Can you work these out from the model? Positions are in its coordinate system, mm. Face numbers are marked on the shaded views. A direction names the side the tool comes from. Round coordinates to 2 decimals unless told otherwise and drop trailing zeros. Order: outer loops, then holes, each group sorted by start corner. A loop starts at its lowest first (then second) coordinate and runs counter-clockwise, first axis right, second up. Notation, with made-up numbers: M 60.5,-3.5 L 108.5,-3.5 A22 cw 108.5,35.5 Z; hole C -4.75,85.5 d8. An arc over 180 degrees is marked long. Answer as a JSON object with one key per item and string values. Group by question number.
```python
from build123d import *

# Parameters (mm, degrees)
SALIENTE_EXTRUIR1_DEPTH = 25.8
CORTAR_EXTRUIR1_REACH   = 53.135
CROQUIS2_R              = 0.986321187
CROQUIS2_W              = 18.5
CROQUIS2_H              = 11.8
CORTAR_EXTRUIR2_DEPTH   = 47.498669213


with BuildPart() as part:
    # Croquis1 → Saliente-Extruir1 (new body)
    with BuildSketch(Plane.XY):
        Polygon((-15.36468389, -0.528688711), (-15.36468389, -1.528688711), (23.08488752, -1.528688711), (23.08488752, -29.783472062), (-25.31094407, -29.783472062), (-25.31094407, -36.701823748), (-24.31094407, -36.701823748), (-24.31094407, -30.783472062), (24.08488752, -30.783472062), (24.08488752, -0.528688711), align=None)
    extrude(amount=SALIENTE_EXTRUIR1_DEPTH)

    # Croquis2 → Cortar-Extruir1 (cut, up to next)
    with BuildSketch(Plane(origin=(0, -0.528688711, 0), x_dir=(1, 0, 0), z_dir=(0, 1, 0)), mode=Mode.PRIVATE) as cortar_extruir1_sk1:
        with Locations(Location((5.43531611, -12.9, 0), (0, 0, 180))):
            Circle(CROQUIS2_R)
    cortar_extruir1_tool1 = extrude(cortar_extruir1_sk1.sketch, amount=-CORTAR_EXTRUIR1_REACH, mode=Mode.PRIVATE) & part.part
    # Croquis2 → Cortar-Extruir1 (cut, up to next)
    with BuildSketch(Plane(origin=(0, -0.528688711, 0), x_dir=(1, 0, 0), z_dir=(0, 1, 0)), mode=Mode.PRIVATE) as cortar_extruir1_sk2:
        with Locations((-6.11468389, -12.9)):
            Rectangle(CROQUIS2_W, CROQUIS2_H)
    cortar_extruir1_tool2 = extrude(cortar_extruir1_sk2.sketch, amount=-CORTAR_EXTRUIR1_REACH, mode=Mode.PRIVATE) & part.part
    add(cortar_extruir1_tool1.solids().sort_by_distance((5.435316, -0.528689, 12.9))[0], mode=Mode.SUBTRACT)
    add(cortar_extruir1_tool2.solids().sort_by_distance((-6.114684, -0.528689, 12.9))[0], mode=Mode.SUBTRACT)

    # Croquis3 → Cortar-Extruir2 (cut, through all)
    with BuildSketch(Plane(origin=(0, -29.783472062, 0), x_dir=(1, 0, 0), z_dir=(0, 1, 0))):
        with BuildLine():
            Line((-25.31094407, -1.35), (9.391397529, -1.35))
            ThreePointArc((9.391397529, -1.35), (13.99905593, -12.9), (9.391397529, -24.45))
            Line((9.391397529, -24.45), (-25.31094407, -24.45))
            Line((-25.31094407, -24.45), (-25.31094407, -1.35))
        make_face()
    extrude(amount=-CORTAR_EXTRUIR2_DEPTH, mode=Mode.SUBTRACT)


solid = part.part
```
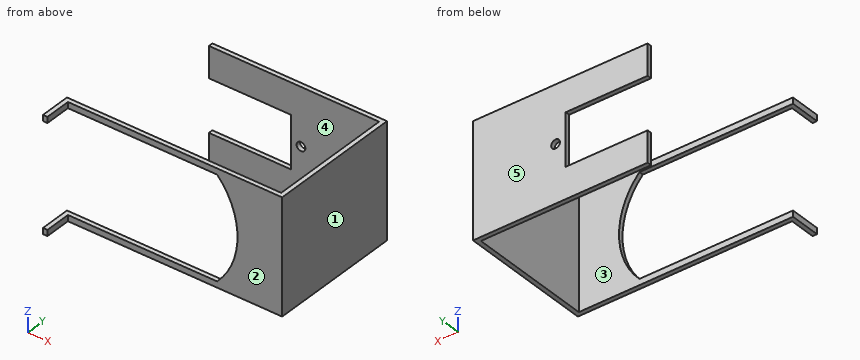
1) Which directions (+Z, -Z, +X, -X, +Y, -Y) give clear straight access to the entire face, cutting with the end or side of a thin tool? Please do the marked faces 4 and 5.
2) For pin 1 (6 mm diameter, centred on x = 6.5, z = 3, fed in from -Y); pin 2 (5.5 mm diameter, centred on x = -1.5, y = -34.5, fed in from +Z); pin 3 (0.7 mm diameter, centred on y = -34, z = 25, fed in from +X); pin 4 (0.8 mm diameter, centred on y = -1, z = 2.5, fed in from -X), each with a flat end and sliding along its axis, tell me the tip position at first contact or that it passes through.
3) If we section it at D-D on x = 12: Write out the boundary of the cut face in (y, z).
4) If we section it at C-C on x = -8.5: Write out the boundary of the cut face in (y, z).
5) I need wall thicknesses on line 1 along Y through (x, z) = (20, 14.75); line 2 along X through (y, z) = (-25, 14.5); line 3 along Y through (x, z) = (-5, 1.5). Which ranges of each line are inside material? Lowest first, please.
6) We'd pull the mould along Y, two halves only. Please class the marked faces 1, 2 and 3: +Y half, -Y half, draft (parallel to the pull), parting line (faces both ways), or undercut.
7) If we section it at A-A on z = 12.9: Write out the boundary of the cut face in (x, y), plus the area to 3 significant figures.
8) If we section it at B-B on x = 17.5: Write out the boundary of the cut face in (y, z), plus the area to 3 significant figures.
Findings:
{
 "1": {"face 4": "+Z, -Z, -X", "face 5": "+Z, -Z, +X, -X, +Y"},
 "2": {"pin 1": "stops at y = -30.78", "pin 2": "passes through", "pin 3": "stops at x = -24.31", "pin 4": "stops at x = -15.36"},
 "3": {"outline": "M -30.78,0 L -29.78,0 L -29.78,4.96 L -30.78,4.96 Z; M -30.78,20.84 L -29.78,20.84 L -29.78,25.8 L -30.78,25.8 Z; M -1.53,0 L -0.53,0 L -0.53,25.8 L -1.53,25.8 Z"},
 "4": {"outline": "M -30.78,0 L -29.78,0 L -29.78,1.35 L -30.78,1.35 Z; M -30.78,24.45 L -29.78,24.45 L -29.78,25.8 L -30.78,25.8 Z; M -1.53,0 L -0.53,0 L -0.53,7 L -1.53,7 Z; M -1.53,18.8 L -0.53,18.8 L -0.53,25.8 L -1.53,25.8 Z"},
 "5": {"line 1": "y = -30.78 to -29.78, -1.53 to -0.53", "line 2": "x = 23.08 to 24.08", "line 3": "y = -1.53 to -0.53"},
 "6": {"face 1": "draft", "face 2": "-Y half", "face 3": "undercut"},
 "7": {"outline": "M 3.14,-1.53 L 4.45,-1.53 L 4.45,-0.53 L 3.14,-0.53 Z; M 6.42,-1.53 L 23.08,-1.53 L 23.08,-29.78 L 14,-29.78 L 14,-30.78 L 24.08,-30.78 L 24.08,-0.53 L 6.42,-0.53 Z", "area": "57.3 mm^2"},
 "8": {"outline": "M -30.78,0 L -29.78,0 L -29.78,25.8 L -30.78,25.8 Z; M -1.53,0 L -0.53,0 L -0.53,25.8 L -1.53,25.8 Z", "area": "51.6 mm^2"}
}
